Check sheet for the modelled part. Datum: model origin and axes. Units: mm. A direction names the side the tool comes from. Round coordinates to 2 decimals unless told otherwise and drop trailing zeros. Loops run counter-clockwise (first coordinate to the right, second up) from the corner with the lowest first, then second, coordinate; pieces in that order, holes last. Notation, with made-up numbers: (34.25, 89.25) - (57.25, 89.25) arc R29 ccw to (57.25, 117.25) - close; hole circle Ø3 at (9.25, 33). An arc over 180 degrees is marked (long way). Return JSON: item names as keys, results as strings.
from build123d import *

# Parameters (mm, degrees)
SKETCH1_W           = 8
SKETCH1_H           = 7
BOSS_EXTRUDE1_DEPTH = 192
SKETCH2_W           = 5
SKETCH2_H           = 3
CUT_EXTRUDE1_DEPTH  = 192
BOSS_EXTRUDE2_DEPTH = 3


with BuildPart() as part:
    # Sketch1 → Boss-Extrude1 (new body)
    with BuildSketch(Plane.XY):
        Rectangle(SKETCH1_W, SKETCH1_H)
    extrude(amount=BOSS_EXTRUDE1_DEPTH)

    # Sketch2 → Cut-Extrude1 (cut)
    with BuildSketch(Plane.XY.offset(192)):
        with Locations((-1.5, 0)):
            Rectangle(SKETCH2_W, SKETCH2_H)
    extrude(amount=-CUT_EXTRUDE1_DEPTH, mode=Mode.SUBTRACT)

    # Sketch3 → Boss-Extrude2 (add)
    with BuildSketch(Plane(origin=(4, 0, 0), x_dir=(0, 0, -1), z_dir=(1, 0, 0))):
        Polygon((-192, -3.5), (0, -40.821019354), (0, -3.5), (0, 3.5), (-192, 3.5), align=None)
    extrude(amount=BOSS_EXTRUDE2_DEPTH)


solid = part.part
Q1. Sectioned sample at D-D (y = -32). Enter the section's corners in (x, z), plus the area to 3 significant figures.
Answer key:
{"outline": "(4, 0) - (7, 0) - (7, 45.38) - (4, 45.38) - close", "area": "136 mm²"}
Q2. Sectioned sample at B-B (y = -23). Enter the section's corners in (x, z).
Answer key:
{"outline": "(4, 0) - (7, 0) - (7, 91.68) - (4, 91.68) - close"}
Q3. Sectioned sample at A-A (z = 42). Enter the section's corners in (x, y), plus the area to 3 significant figures.
Answer key:
{"outline": "(-4, -3.5) - (4, -3.5) - (4, -32.66) - (7, -32.66) - (7, 3.5) - (-4, 3.5) - (-4, 1.5) - (1, 1.5) - (1, -1.5) - (-4, -1.5) - close", "area": "149 mm²"}
Q4. Scan lines: probe 1 along Y at (x, z) = (-2.25, 65); probe 2 along X at (y, z) = (-9, 107.5); probe 3 along X at (y, z) = (0.5, 85). Record each from-to range of solid material in increasing order. Write a range as [from, to].
Answer key:
{"probe 1": "y = [-3.5, -1.5], [1.5, 3.5]", "probe 2": "x = [4, 7]", "probe 3": "x = [1, 7]"}
Q5. Sectioned sample at C-C (z = 108). Enter the section's corners in (x, y), plus the area to 3 significant figures.
Answer key:
{"outline": "(-4, -3.5) - (4, -3.5) - (4, -19.83) - (7, -19.83) - (7, 3.5) - (-4, 3.5) - (-4, 1.5) - (1, 1.5) - (1, -1.5) - (-4, -1.5) - close", "area": "111 mm²"}
Q6. Draft check along Y on faces 4 (the face through (-2, -1.5, 97)), 5 (the face through (1, 3.5, 95)), 6 (the face through (-2, 1.5, 97)), 7 (the face through (0, -3.5, 95)). Enter one of: released by +Y, released by -Y, zero draft, split by the parting line, or undercut.
Answer key:
{"face 4": "undercut", "face 5": "released by +Y", "face 6": "undercut", "face 7": "released by -Y"}
Q7. Tool access check on faces 1 (the face through (5.48, -21.9, 97.34)), 2 (the face through (4, -14, 55)), 3 (the face through (1, 0, 97)). Record the directions out of +Z, -Z, +X, -X, +Y, -Y that give a thin tool (end or side, any length) a straight path to the whole face; none if there is none.
Answer key:
{"face 1": "+Z, +X, -X, -Y", "face 2": "+Z, -Z, -X, -Y", "face 3": "+Z, -Z, -X"}
Q8. Depth check by flat-ended pin: P1, Ø5.5, axis at x = -2, z = 139.5, coming from the -Y side; P2, Ø0.9, axis at y = 0, z = 103.5, coming from the -X side; P3, Ø1.5, axis at y = -11.5, z = 113, coming from the -X side; P4, Ø10, axis at y = -23.5, z = 132, coming from the -X side. Enter the tip coordinate at first touch or a pass-through.
Answer key:
{"P1": "stops at y = -3.5", "P2": "stops at x = 1", "P3": "stops at x = 4", "P4": "passes through"}
